The figure shows three views and two pictorial views of one solid part (mm, origin at its lowest corner). Answer the questions. Coordinates: 2 decimals unless noted, no trailing zeros. Order: outer loops, then holes, each group sorted by start corner. A loop starts at its lowest first (then second) coordinate and runs counter-clockwise, first axis right, second up. Notation, with made-up numbers: M -29,-35 L 25,-35 A13 ccw 25,-24 Z; hole C 47.5,72 d3. An arc over 180 degrees is marked long. Answer in a Markdown table with one row per item. Add a question column.
Item 1: The part is cut by section A-A (x = 63.5). Write down the section's boundary in (y, z), then the cut area to 3 significant figures.
Item 2: The part is cut by section B-B (y = 89.4). Write down the section's boundary in (x, z), then the cut area to 3 significant figures.
Item 3: The part is cut by section C-C (x = 82.5). Write down the section's boundary in (y, z).
Item 4: The part is cut by section D-D (z = 2.5). State how many separate pieces and enclosed holes the cut face has, then the cut area to 3 significant figures.
Item 5: Consider line 1 (X direction, y = 89.4, z = 2.75); line 2 (Y direction, x = 98.2, z = 3.5); line 3 (X direction, y = 108, z = 2.75). Determine where each line is inside the solid, lowest interval first. Write a range as from..to.
Item 6: Flat-ended cylindrical pins translate along their axes: pin 1 Ø13.5 at (x, y) = (27.5, 57.4) entering from +Z; pin 2 Ø2 at (x, y) = (8, 10) entering from +Z. Find the tip coordinate at first contact, or state that the pin passes through.
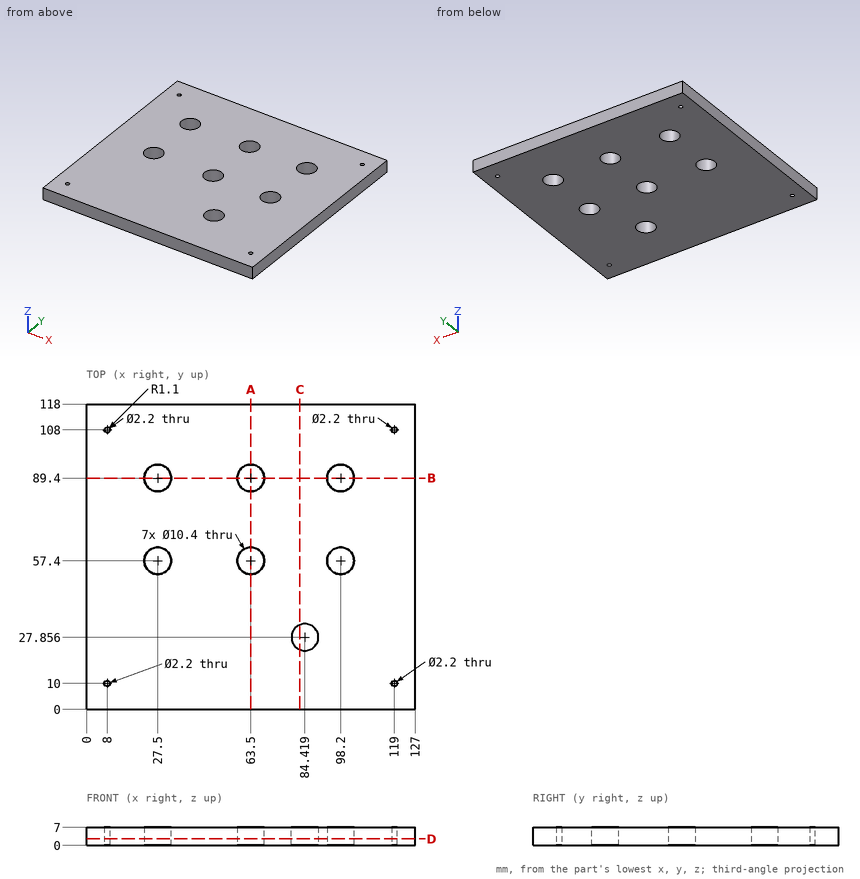
Reply:
| question | item | result |
|---|---|---|
| 1 | outline | M 0,0 L 52.2,0 L 52.2,7 L 0,7 Z; M 62.6,0 L 84.2,0 L 84.2,7 L 62.6,7 Z; M 94.6,0 L 118,0 L 118,7 L 94.6,7 Z |
| 1 | area | 680 mm2 |
| 2 | outline | M 0,0 L 22.3,0 L 22.3,7 L 0,7 Z; M 32.7,0 L 58.3,0 L 58.3,7 L 32.7,7 Z; M 68.7,0 L 93,0 L 93,7 L 68.7,7 Z; M 103.4,0 L 127,0 L 127,7 L 103.4,7 Z |
| 2 | area | 671 mm2 |
| 3 | outline | M 0,0 L 23.02,0 L 23.02,7 L 0,7 Z; M 32.69,0 L 118,0 L 118,7 L 32.69,7 Z |
| 4 | separate pieces | 1 |
| 4 | enclosed holes | 11 |
| 4 | area | 14,400 mm2 |
| 5 | line 1 | x = 0..22.3, 32.7..58.3, 68.7..93, 103.4..127 |
| 5 | line 2 | y = 0..52.2, 62.6..84.2, 94.6..118 |
| 5 | line 3 | x = 0..6.9, 9.1..117.9, 120.1..127 |
| 6 | pin 1 | stops at z = 7 |
| 6 | pin 2 | passes through |
